```python
from build123d import *

# Parameters (mm, degrees)
SKETCH1_W           = 80
SKETCH1_H           = 57.5
BOSS_EXTRUDE1_DEPTH = 3.5
SKETCH3_R           = 1
BOSS_EXTRUDE2_DEPTH = 0.5


with BuildPart() as part:
    # Sketch1 → Boss-Extrude1 (new, symmetric)
    with BuildSketch(Plane.XY):
        Rectangle(SKETCH1_W, SKETCH1_H)
    extrude(amount=BOSS_EXTRUDE1_DEPTH, both=True)

    # Sketch3 → Boss-Extrude2 (add, symmetric)
    # profile 1 of 4: a face of its own
    with BuildSketch(Plane.XY):
        with BuildLine():
            Line((40, 19), (43, 19))
            ThreePointArc((43, 19), (46, 16), (43, 13))
            Line((43, 13), (40, 13))
            Line((40, 13), (40, 19))
        make_face()
        with Locations((43, 16)):
            Circle(SKETCH3_R, mode=Mode.SUBTRACT)
    # profile 2 of 4: a face of its own
    with BuildSketch(Plane.XY):
        with BuildLine():
            Line((43, -19), (40, -19))
            Line((40, -19), (40, -13))
            Line((40, -13), (43, -13))
            ThreePointArc((43, -13), (46, -16), (43, -19))
        make_face()
        with Locations((43, -16)):
            Circle(SKETCH3_R, mode=Mode.SUBTRACT)
    # profile 3 of 4: a face of its own
    with BuildSketch(Plane.XY):
        with BuildLine():
            Line((-43, 19), (-40, 19))
            Line((-40, 19), (-40, 13))
            Line((-40, 13), (-43, 13))
            ThreePointArc((-43, 13), (-46, 16), (-43, 19))
        make_face()
        with Locations((-43, 16)):
            Circle(SKETCH3_R, mode=Mode.SUBTRACT)
    # profile 4 of 4: a face of its own
    with BuildSketch(Plane.XY):
        with BuildLine():
            Line((-43, -13), (-40, -13))
            Line((-40, -13), (-40, -19))
            Line((-40, -19), (-43, -19))
            ThreePointArc((-43, -19), (-46, -16), (-43, -13))
        make_face()
        with Locations((-43, -16)):
            Circle(SKETCH3_R, mode=Mode.SUBTRACT)
    extrude(amount=BOSS_EXTRUDE2_DEPTH, both=True)


solid = part.part
```
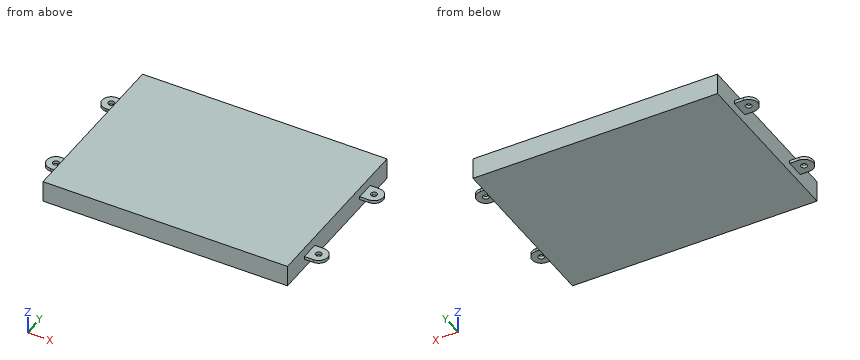
Check sheet for the modelled part. Datum: model origin and axes. Units: mm. Coordinates: 2 decimals unless noted, no trailing zeros. Loops run counter-clockwise (first coordinate to the right, second up) from the corner with the lowest first, then second, coordinate; pieces in that order, holes last.
1) Material ranges on probe 1 along Y at (x, z) = (43, 0.3); probe 2 along X at (y, z) = (-18, -1.75), recorded low to high.
2) Sectioned sample at C-C (y = -4.5). Record the boundary of the cut face in (x, z).
3) Sectioned sample at B-B (z = 1.5). Record the boundary of the cut face in (x, y), and give its area (3 significant figures).
4) Gauge pin test, flat ends, axial feed: pin 1 (1.5 mm diameter, centred on y = -6, z = 2.5, fed in from -X); pin 2 (3 mm diameter, centred on x = 43, y = -16, fed in from -Z); pin 3 (0.8 mm diameter, centred on x = 42, z = 0, fed in from +Y). Record the tip position at first contact, or that the pin passes through.
5) Sectioned sample at A-A (y = 16). Record the boundary of the cut face in (x, z).
Check sheet entries:
1. probe 1: y = -19 to -17, -15 to -13, 13 to 15, 17 to 19
1. probe 2: x = -40 to 40
2. outline: (-40, -3.5) - (40, -3.5) - (40, 3.5) - (-40, 3.5) - close
3. outline: (-40, -28.75) - (40, -28.75) - (40, 28.75) - (-40, 28.75) - close
3. area: 4,600 mm2
4. pin 1: stops at x = -40
4. pin 2: stops at z = -0.5
4. pin 3: stops at y = 19
5. outline: (-46, -0.5) - (-44, -0.5) - (-44, 0.5) - (-46, 0.5) - close; (-42, -0.5) - (-40, -0.5) - (-40, -3.5) - (40, -3.5) - (40, -0.5) - (42, -0.5) - (42, 0.5) - (40, 0.5) - (40, 3.5) - (-40, 3.5) - (-40, 0.5) - (-42, 0.5) - close; (44, -0.5) - (46, -0.5) - (46, 0.5) - (44, 0.5) - close
